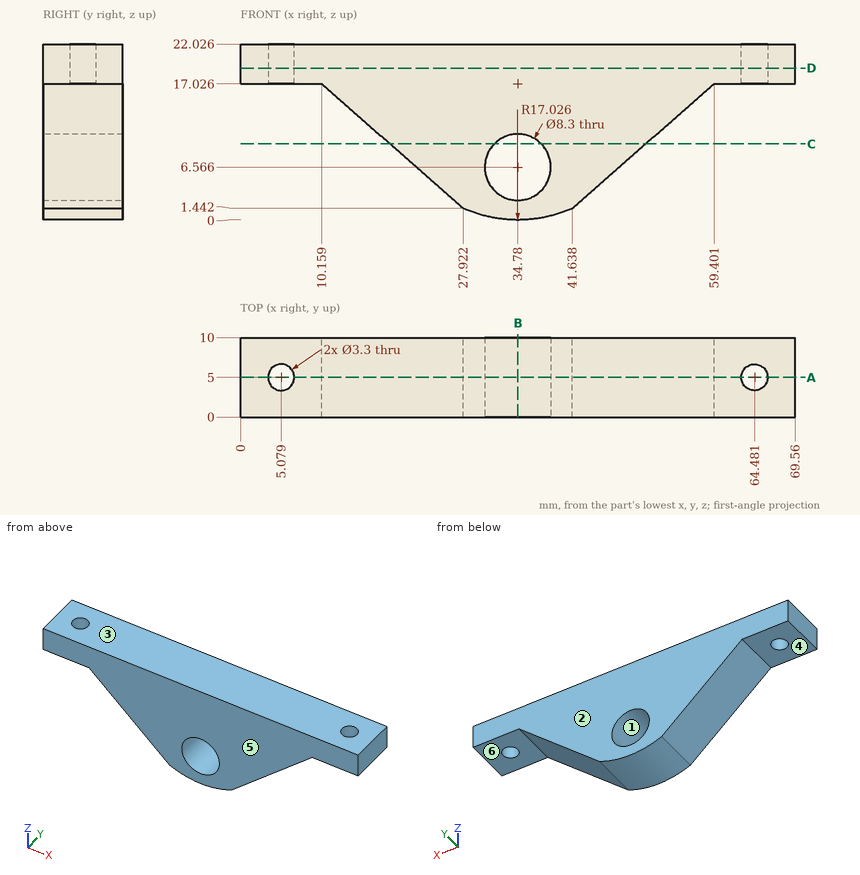
Answer from the drawing. Dimensions are ordinates in mm from the lowest x, y and z of the part. A direction names the side the tool comes from. Coordinates: 2 decimals unless noted, no trailing zeros. Write each loop counter-clockwise with the first axis right and the second up, starting at its lowest first coordinate (ties: lowest second). Pieces come first, ordered by that corner, then holes. Notation, with made-up numbers: (49, 16.5) - (99, 16.5) arc R31 ccw to (99, 48.5) - close; hole circle Ø11 at (21.25, 36.25). An arc over 180 degrees is marked (long way). Return JSON: item names as keys, results as strings. Group by question number.
Q1. Flat-ended cylindrical pins translate along their axes: pin 1 Ø8 at (x, z) = (58, 14.5) entering from +Y; pin 2 Ø6.5 at (x, z) = (34.78, 6.57) entering from +Y; pin 3 Ø5 at (x, y) = (62.5, 5) entering from -Z; pin 4 Ø2 at (y, z) = (6.5, 4.5) entering from -X (1 decimal). Find the tip coordinate at first contact, or state that the pin passes through.
Q2. The part is cut by section C-C on z = 9.5. Write down the section's boundary in (x, y) (1 decimal), and give its area (3 significant figures).
Q3. The part is cut by section D-D on z = 19. Write down the section's boundary in (x, y).
Q4. For a pull along Z with two mould halves and no side action, classify the marked faces 1, 2, 3 and 4 as +Z half, -Z half, draft (parallel to the pull), parting line (faces both ways), or undercut.
Q5. Which of the six approach directions +Z, -Z, +X, -X, +Y, -Y give full straight-line access (tool end or side, diameter ignored) to the marked faces 5 and 6?
Q6. Find the intervals of material crossed by line 1 along X through (y, z) = (4, 18.75) (1 decimal); line 2 along X through (y, z) = (9, 9.25) (1 decimal); line 3 along Z through (x, y) = (63.5, 1.5), in increasing order. Write a range as [from, to].
Q7. The part is cut by section B-B on x = 34.78. Write down the section's boundary in (y, z), and give its area (3 significant figures).
Q8. The part is cut by section A-A on y = 5. Write down the section's boundary in (x, z).
Evaluation:
{
 "1": {"pin 1": "stops at y = 10", "pin 2": "passes through", "pin 3": "stops at z = 17.03", "pin 4": "stops at x = 23.3"},
 "2": {"outline": "(18.7, 0) - (31.8, 0) - (31.8, 10) - (18.7, 10) - close; (37.7, 0) - (50.8, 0) - (50.8, 10) - (37.7, 10) - close", "area": "262 mm2"},
 "3": {"outline": "(0, 0) - (69.56, 0) - (69.56, 10) - (0, 10) - close; hole circle Ø3.3 at (5.08, 5); hole circle Ø3.3 at (64.48, 5)"},
 "4": {"face 1": "undercut", "face 2": "draft", "face 3": "+Z half", "face 4": "-Z half"},
 "5": {"face 5": "+Z, -Z, +X, -X, -Y", "face 6": "-Z, +X, +Y, -Y"},
 "6": {"line 1": "x = [0, 3.8], [6.4, 63.2], [65.8, 69.6]", "line 2": "x = [19, 31.6], [37.9, 50.5]", "line 3": "z = [17.03, 22.03]"},
 "7": {"outline": "(0, 0) - (10, 0) - (10, 2.42) - (0, 2.42) - close; (0, 10.72) - (10, 10.72) - (10, 22.03) - (0, 22.03) - close", "area": "137 mm2"},
 "8": {"outline": "(0, 17.03) - (3.43, 17.03) - (3.43, 22.03) - (0, 22.03) - close; (6.73, 17.03) - (10.16, 17.03) - (27.92, 1.44) arc R17.03 ccw to (41.64, 1.44) - (59.4, 17.03) - (62.83, 17.03) - (62.83, 22.03) - (6.73, 22.03) - close; (66.13, 17.03) - (69.56, 17.03) - (69.56, 22.03) - (66.13, 22.03) - close; hole circle Ø8.3 at (34.78, 6.57)"}
}
